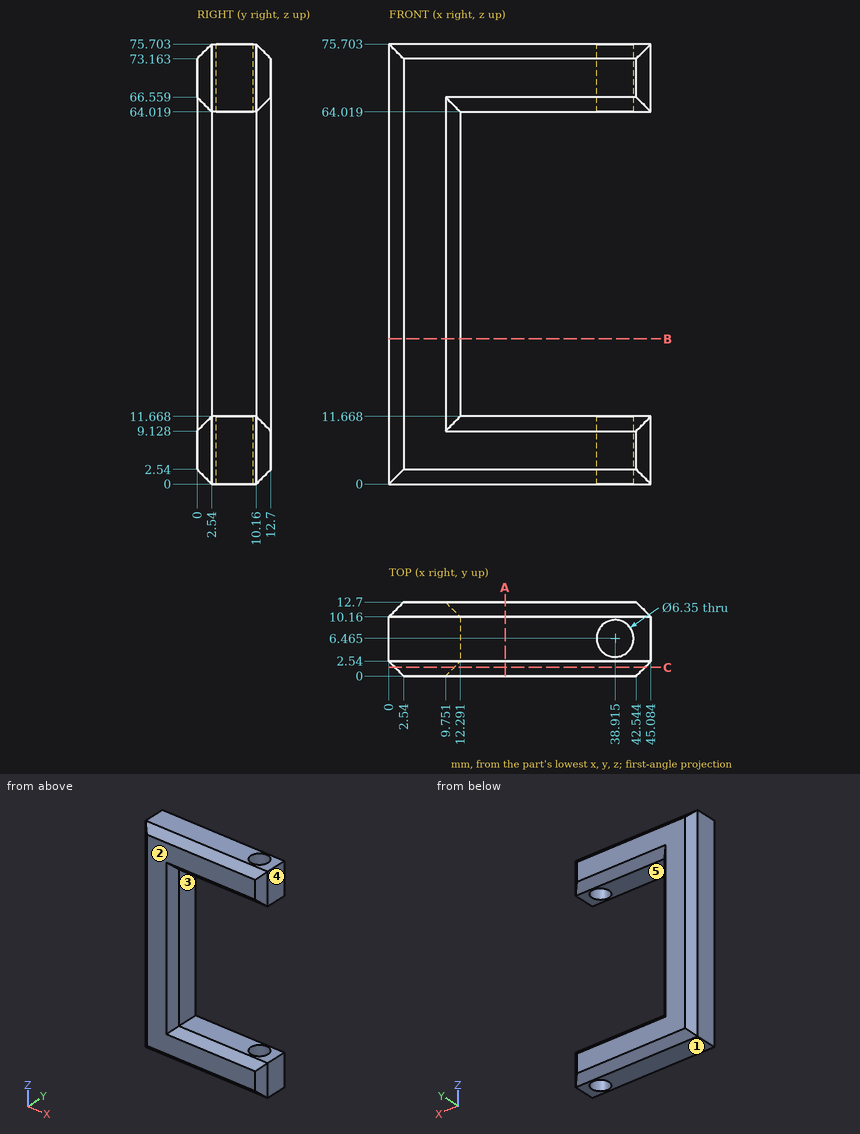
For this review, use the dimensioned drawing (mm, ordinates from the lowest corner) and the shaded views. A direction names the side the tool comes from. Coordinates: 2 decimals unless noted, no trailing zeros. Order: outer loops, then holes, each group sorted by start corner. A loop starts at its lowest first (then second) coordinate and runs counter-clockwise, first axis right, second up. Notation, with made-up numbers: (1, 5) - (43, 5) arc R14 ccw to (43, 17) - close; hole circle Ø7 at (-20.75, -9.75). An arc over 180 degrees is marked (long way). Answer as a JSON object with one key per item and string values. Group by question number.
1. For probe 1 along Z at (x, y) = (20, 8); probe 2 along X at (y, z) = (9.5, 27); probe 3 along X at (y, z) = (9, 8.5) (1 decimal), list the stretches that pass through material, from the lowest coordinate up.
2. We need section B-B on z = 25. State the section outline as (x, y) points, then the cut area to 3 significant figures.
3. The part is to be moulded in two halves that separate along Z. For the marked faces 1, 2 and 3, say which applies: pulls with the +Z half, pulls with the -Z half, needs draft (parallel to the pull), parting line crosses it, or undercut.
4. For the marked faces 4 and 5, list the 3-axis set-ups (+Z, -Z, +X, -X, +Y, -Y) from which the entire face can be reached by the end or side of a thin tool; tool diameter is ignored.
5. We need section A-A on x = 20. State the section outline as (y, z) points, then the cut area to 3 significant figures.
6. Clearance check with a flat-ended pin moving along its axis: P1, Ø6, axis at x = 37, y = 8, coming from the +Z side. State where the tip first meets the part, or that it passes through.
7. We need section C-C on y = 1.5. State the section outline as (x, z) points, then the cut area to 3 significant figures.
Final values:
{
 "1": {"probe 1": "0 to 11.67, 64.02 to 75.7", "probe 2": "0 to 12.29", "probe 3": "0 to 37, 40.8 to 45.1"},
 "2": {"outline": "(0, 2.54) - (2.54, 0) - (9.75, 0) - (12.29, 2.54) - (12.29, 10.16) - (9.75, 12.7) - (2.54, 12.7) - (0, 10.16) - close", "area": "143 mm²"},
 "3": {"face 1": "pulls with the -Z half", "face 2": "needs draft", "face 3": "undercut"},
 "4": {"face 4": "+Z, -Z, +X, +Y, -Y", "face 5": "+X, +Y, -Y"},
 "5": {"outline": "(0, 2.54) - (2.54, 0) - (10.16, 0) - (12.7, 2.54) - (12.7, 9.13) - (10.16, 11.67) - (2.54, 11.67) - (0, 9.13) - close; (0, 66.56) - (2.54, 64.02) - (10.16, 64.02) - (12.7, 66.56) - (12.7, 73.16) - (10.16, 75.7) - (2.54, 75.7) - (0, 73.16) - close", "area": "271 mm²"},
 "6": {"P1": "z = 75.7"},
 "7": {"outline": "(1.04, 1.04) - (44.04, 1.04) - (44.04, 10.63) - (11.25, 10.63) - (11.25, 65.06) - (44.04, 65.06) - (44.04, 74.66) - (1.04, 74.66) - close", "area": "1,380 mm²"}
}
